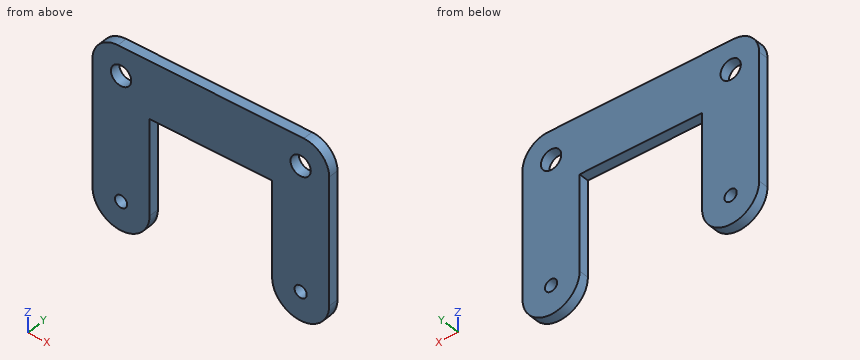
```python
from build123d import *

# Parameters (mm, degrees)
SKETCH1_R           = 4
SKETCH1_R_2         = 11.25
SKETCH1_R_3         = 2.4
BOSS_EXTRUDE1_DEPTH = 4
FILLET1_R           = 10


with BuildPart() as part:
    # Sketch1 → Boss-Extrude1 (new body)
    with BuildSketch(Plane(origin=(0, 0, 0), x_dir=(1, 0, 0), z_dir=(0, 1, 0))):
        with BuildLine():
            Line((-24.125, -37.5), (-24.125, 0))
            ThreePointArc((-24.125, 0), (-35.375, -11.25), (-46.625, 0))
            Line((-46.625, 0), (-46.625, -60))
            Line((-46.625, -60), (46.625, -60))
            Line((46.625, -60), (46.625, 0))
            ThreePointArc((46.625, 0), (35.375, -11.25), (24.125, 0))
            Line((24.125, 0), (24.125, -37.5))
            Line((24.125, -37.5), (-24.125, -37.5))
        make_face()
        with Locations((-35.375, -48.75)):
            Circle(SKETCH1_R, mode=Mode.SUBTRACT)
        with Locations((35.375, -48.75)):
            Circle(SKETCH1_R, mode=Mode.SUBTRACT)
        with Locations((-35.375, 0)):
            Circle(SKETCH1_R_2)
        with Locations((-35.375, 0)):
            Circle(SKETCH1_R_3, mode=Mode.SUBTRACT)
        with Locations((35.375, 0)):
            Circle(SKETCH1_R_2)
        with Locations((35.375, 0)):
            Circle(SKETCH1_R_3, mode=Mode.SUBTRACT)
    extrude(amount=BOSS_EXTRUDE1_DEPTH)

    # Fillet1
    fillet1_edges = [part.edges().sort_by_distance(p)[0] for p in [
        (46.625, 2, 60),
        (-46.625, 2, 60),
    ]]
    fillet(fillet1_edges, radius=FILLET1_R)


solid = part.part
```
The listing builds one solid part. Answer for the finished solid, in the listing's coordinates (mm). Give positions to 0.01 mm unless a question says otherwise; leave off trailing zeros. Loops run counter-clockwise (first coordinate to the right, second up) from the corner with the lowest first, then second, coordinate; pieces in that order, holes last. Notation, with made-up numbers: M -10,-38 L 40,-38 A16 cw 40,-11 Z; hole C 51,13.25 d7. An arc over 180 degrees is marked long. One line per item, written item: value.
1. Section D-D on x = 17.5 is taken. Determine the outline of the cut face in (y, z).
Found:
outline: M 0,37.5 L 4,37.5 L 4,60 L 0,60 Z
2. Section C-C on y = 2.1 is taken. Determine the outline of the cut face in (x, z) (3 decimals).
Found:
outline: M -46.625,0 A11.25 ccw -24.125,0 L -24.125,37.5 L 24.125,37.5 L 24.125,0 A11.25 ccw 46.625,0 L 46.625,50 A10 ccw 36.625,60 L -36.625,60 A10 ccw -46.625,50 Z; hole C -35.375,48.75 d8; hole C -35.375,0 d4.8; hole C 35.375,48.75 d8; hole C 35.375,0 d4.8
3. Find the intervals of material crossed by probe 1 along Z at (x, y) = (-36.5, 1.4); probe 2 along Z at (x, y) = (-35.5, 2.05); probe 3 along X at (y, z) = (0.4, 21) (3 decimals), in increasing order.
Found:
probe 1: -11.19 to -2.12, 2.12 to 44.91, 52.59 to 60
probe 2: -11.25 to -2.4, 2.4 to 44.75, 52.75 to 60
probe 3: -46.625 to -24.125, 24.125 to 46.625
4. Section A-A on z = 36 is taken. Determine the outline of the cut face in (x, y) (3 decimals).
Found:
outline: M -46.625,0 L -24.125,0 L -24.125,4 L -46.625,4 Z; M 24.125,0 L 46.625,0 L 46.625,4 L 24.125,4 Z
5. Section B-B on z = 48.75 is taken. Determine the outline of the cut face in (x, y) (3 decimals).
Found:
outline: M -46.625,0 L -39.375,0 L -39.375,4 L -46.625,4 Z; M -31.375,0 L 31.375,0 L 31.375,4 L -31.375,4 Z; M 39.375,0 L 46.625,0 L 46.625,4 L 39.375,4 Z
